Build history of the part. All positions in model axes, mm. A direction names the side the tool comes from. Coordinates: 2 decimals unless noted, no trailing zeros. Order: outer loops, then holes, each group sorted by start corner. A loop starts at its lowest first (then second) coordinate and runs counter-clockwise, first axis right, second up. Notation, with made-up numbers: (23.5, -12) - (29.5, -12) arc R22 ccw to (29.5, 13) - close; hole circle Ø5 at (53.5, 83). An arc over 180 degrees is marked (long way). One line per item, written item: value.
from build123d import *

# Parameters (mm, degrees)
EXTRUDE_1_DEPTH     = 4
SKETCH_3_W          = 43.235473071
SKETCH_3_H          = 2
EXTRUDE_2_DEPTH     = 20
SKETCH_4_W          = 43.235473071
SKETCH_4_H          = 21
EXTRUDE_3_DEPTH     = 15
SKETCH_8_W          = 3
SKETCH_8_H          = 10
EXTRUDE_4_DEPTH     = 10
SKETCH_10_R         = 1.4
CUT_EXTRUDE_1_DEPTH = 83
SKETCH_11_W         = 3
SKETCH_11_H         = 90
EXTRUDE_5_DEPTH     = 80
SKETCH_12_W         = 72.707770749
SKETCH_12_H         = 25
EXTRUDE_6_DEPTH     = 5
SKETCH_13_W         = 46
SKETCH_13_H         = 20
CUT_EXTRUDE_2_DEPTH = 4
CUT_EXTRUDE_3_REACH = 123
SKETCH_14_W         = 15
SKETCH_14_H         = 5
SKETCH_15_R         = 1.2
CUT_EXTRUDE_4_DEPTH = 10


with BuildPart() as part:
    # 草圖1 → 填料-伸長1 (new body)
    with BuildSketch(Plane.XY):
        Polygon((-37.5, 45), (-35, 45), (-35, 80), (15, 80), (15, 45), (37.5, 45), (37.5, -45), (-37.5, -45), align=None)
    extrude(amount=EXTRUDE_1_DEPTH)

    # 草圖3 → 填料-伸長2 (add)
    with BuildSketch(Plane.XY.offset(4)):
        with Locations((-6.617736535, 56)):
            Rectangle(SKETCH_3_W, SKETCH_3_H)
        with Locations((-6.617736535, 79)):
            Rectangle(SKETCH_3_W, SKETCH_3_H)
    extrude(amount=EXTRUDE_2_DEPTH)

    # 草圖4 → 填料-伸長3 (add)
    with BuildSketch(Plane.XY.offset(4)):
        with Locations((-6.617736535, 67.5)):
            Rectangle(SKETCH_4_W, SKETCH_4_H)
    extrude(amount=EXTRUDE_3_DEPTH)

    # 草圖8 → 填料-伸長4 (add)
    with BuildSketch(Plane(origin=(0, 0, 0), x_dir=(-1, 0, 0), z_dir=(0, 0, -1))):
        with Locations((-36, 40)):
            Rectangle(SKETCH_8_W, SKETCH_8_H)
        with Locations((36, 40)):
            Rectangle(SKETCH_8_W, SKETCH_8_H)
        with Locations((36, -40)):
            Rectangle(SKETCH_8_W, SKETCH_8_H)
        with Locations((-36, -40)):
            Rectangle(SKETCH_8_W, SKETCH_8_H)
    extrude(amount=EXTRUDE_4_DEPTH)

    # 草圖10 → 除料-伸長1 (cut)
    with BuildSketch(Plane(origin=(37.5, 0, 0), x_dir=(0, 0, -1), z_dir=(1, 0, 0))):
        with Locations((5, 40)):
            Circle(SKETCH_10_R)
        with Locations((5, -40)):
            Circle(SKETCH_10_R)
    extrude(amount=-CUT_EXTRUDE_1_DEPTH, mode=Mode.SUBTRACT)

    # 草圖11 → 填料-伸長5 (add)
    with BuildSketch(Plane.XY.offset(4)):
        with Locations((-36, 0)):
            Rectangle(SKETCH_11_W, SKETCH_11_H)
        with Locations((36, 0)):
            Rectangle(SKETCH_11_W, SKETCH_11_H)
    extrude(amount=EXTRUDE_5_DEPTH)

    # 草圖12 → 填料-伸長6 (add)
    with BuildSketch(Plane.XZ.offset(45)):
        with Locations((0.126228768, 61.5)):
            Rectangle(SKETCH_12_W, SKETCH_12_H)
    extrude(amount=-EXTRUDE_6_DEPTH)

    # 草圖13 → 除料-伸長2 (cut)
    with BuildSketch(Plane.XZ.offset(45)):
        with Locations((0, 64)):
            Rectangle(SKETCH_13_W, SKETCH_13_H)
    extrude(amount=-CUT_EXTRUDE_2_DEPTH, mode=Mode.SUBTRACT)

    # 草圖14 → 除料-伸長3 (cut, up to next)
    with BuildSketch(Plane.XZ.offset(41), mode=Mode.PRIVATE) as cut_extrude_3_sk1:
        with Locations((0, 71.5)):
            Rectangle(SKETCH_14_W, SKETCH_14_H)
    cut_extrude_3_tool1 = extrude(cut_extrude_3_sk1.sketch, amount=-CUT_EXTRUDE_3_REACH, mode=Mode.PRIVATE) & part.part
    add(cut_extrude_3_tool1.solids().sort_by_distance((0, -41, 71.5))[0], mode=Mode.SUBTRACT)

    # 草圖15 → 除料-伸長4 (cut)
    with BuildSketch(Plane(origin=(15, 0, 0), x_dir=(0, 0, -1), z_dir=(1, 0, 0))):
        with Locations((-16.1, 72.2)):
            Circle(SKETCH_15_R)
        with Locations((-16.1, 62.8)):
            Circle(SKETCH_15_R)
    extrude(amount=-CUT_EXTRUDE_4_DEPTH, mode=Mode.SUBTRACT)


solid = part.part
1. Probe line 1 along Y through (x, z) = (11.5, 16.1); line 2 along X through (y, z) = (-5, 21.5); line 3 along Y through (x, z) = (-36, -5). List the from-to ranges inside material, lowest first.
Values found:
line 1: y = 55 to 61.6, 64 to 71, 73.4 to 80
line 2: x = -37.5 to -34.5, 34.5 to 37.5
line 3: y = -45 to -41.4, -38.6 to -35, 35 to 38.6, 41.4 to 45
2. Band-saw the part on C-C, the plane y = 40. Give the cut face in (x, z).
Values found:
outline: (-37.5, -10) - (-34.5, -10) - (-34.5, -6.4) - (-37.5, -6.4) - close; (-37.5, -3.6) - (-34.5, -3.6) - (-34.5, 0) - (34.5, 0) - (34.5, -3.6) - (37.5, -3.6) - (37.5, 84) - (34.5, 84) - (34.5, 4) - (-34.5, 4) - (-34.5, 84) - (-37.5, 84) - close; (34.5, -10) - (37.5, -10) - (37.5, -6.4) - (34.5, -6.4) - close
3. 3-axis set-ups, long thin cutter, end or side, ignore diameter. For faces 4 (the face through (-34.5, 41, -3.8)), 5 (the face through (-7, 78, 21)), 6 (the face through (36, 35, -5)), 7 (the face through (23, -43, 64)): which of +Z, -Z, +X, -X, +Y, -Y reach the whole face in a straight line?
Values found:
face 4: -Z, +Y, -Y
face 5: +Z, +X, -X
face 6: -Z, +X, -X
face 7: +Z, -Y
4. Flat gauge pins, fed straight in: P1, Ø3, axis at x = 2.5, y = 6, coming from the -Z side; P2, Ø2, axis at y = -40, z = -5, coming from the -X side (3 decimals); P3, Ø3, axis at y = 72.2, z = 16.1, coming from the +X side; P4, Ø5.5, axis at x = 4, z = 22, coming from the -Y side. Where does each tip first touch, or does it go through?
Values found:
P1: stops at z = 0
P2: passes through
P3: stops at x = 15
P4: stops at y = 55
5. Band-saw the part on B-B, the plane z = 21. Give the cut face in (x, y), and give its area (3 significant figures).
Values found:
outline: (-37.5, -45) - (-34.5, -45) - (-34.5, 45) - (-37.5, 45) - close; (-28.24, 55) - (15, 55) - (15, 57) - (-28.24, 57) - close; (-28.24, 78) - (15, 78) - (15, 80) - (-28.24, 80) - close; (34.5, -45) - (37.5, -45) - (37.5, 45) - (34.5, 45) - close
area: 713 mm2
6. Two-plate mould, pull along Z, no slides. Class faces 1 (the face through (0, -43, 49)), 2 (the face through (-37.5, -1, 36)), 3 (the face through (36, 1, 84)): pulls with the +Z half, pulls with the -Z half, needs draft (parallel to the pull), parting line crosses it, or undercut.
Values found:
face 1: undercut
face 2: needs draft
face 3: pulls with the +Z half
7. Band-saw the part on D-D, the plane x = 29. Give the cut face in (y, z).
Values found:
outline: (-45, 0) - (45, 0) - (45, 4) - (-45, 4) - close; (-45, 49) - (-40, 49) - (-40, 74) - (-45, 74) - close
8. Band-saw the part on A-A, the plane x = 13. Give the cut face in (y, z), and give its area (3 significant figures).
Values found:
outline: (-45, 0) - (80, 0) - (80, 24) - (78, 24) - (78, 19) - (57, 19) - (57, 24) - (55, 24) - (55, 4) - (-45, 4) - close; (-45, 49) - (-40, 49) - (-40, 74) - (-41, 74) - (-41, 54) - (-45, 54) - close; hole circle Ø2.4 at (62.8, 16.1); hole circle Ø2.4 at (72.2, 16.1)
area: 931 mm2
